Here's how the part is built. I have some questions about the finished solid (model axes, mm). Round coordinates to 2 decimals unless told otherwise and drop trailing zeros. Order: outer loops, then holes, each group sorted by start corner. A loop starts at its lowest first (then second) coordinate and runs counter-clockwise, first axis right, second up.
```python
from build123d import *

# Parameters (mm, degrees)
EXTRUDE_2_DEPTH    = 12
CHAMFER_1_SIZE     = 3
HOLE_WIZARD_M6_2_D = 5
F_8_0MM_1_D        = 8


with BuildPart() as part:
    # 草圖2 → 填料-伸長2 (new body)
    with BuildSketch(Plane(origin=(0, 0, 0), x_dir=(1, 0, 0), z_dir=(0, 1, 0))):
        Polygon((0, 86.602540378), (-75, 43.301270189), (-75, -43.301270189), (0, -86.602540378), (75, -43.301270189), (75, 43.301270189), align=None)
    extrude(amount=EXTRUDE_2_DEPTH)

    # 導角1
    chamfer_1_edges = [part.edges().sort_by_distance(p)[0] for p in [
        (-75, 12, 0),
        (-37.5, 12, 64.951905284),
        (37.5, 12, 64.951905284),
        (75, 12, 0),
        (37.5, 12, -64.951905284),
        (-37.5, 12, -64.951905284),
    ]]
    chamfer(chamfer_1_edges, length=CHAMFER_1_SIZE)

    # M6 螺紋孔2 (through all)
    with Locations(Plane(origin=(-65, 12, 37.527767497), x_dir=(0, 0, 1), z_dir=(0, 1, 0))):
        with Locations((0, 0), (-75.055534994, 0), (-112.583302492, 65), (-75.055534994, 130), (-37.527767497, 130), (37.527767498, 65), (0, 130)):
            Hole(HOLE_WIZARD_M6_2_D / 2)

    # Ø8.0mm 定位孔1 (through all)
    with Locations(Plane(origin=(-65, 12, 0), x_dir=(0, 0, 1), z_dir=(0, 1, 0))):
        with Locations((0, 0), (56.5, 32.5), (56.5, 97.5), (-56.5, 97.5), (-56.5, 32.5)):
            Hole(F_8_0MM_1_D / 2)


solid = part.part
```
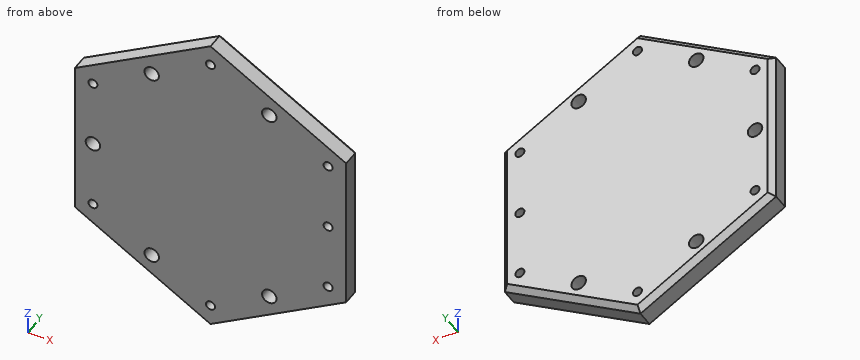
1. If we section it at A-A, the plane z = 0: Write out the boundary of the cut face in (x, y).
Evaluation:
outline: (-75, 0) - (-69, 0) - (-69, 12) - (-72, 12) - (-75, 9) - close; (-61, 0) - (62.5, 0) - (62.5, 12) - (-61, 12) - close; (67.5, 0) - (75, 0) - (75, 9) - (72, 12) - (67.5, 12) - close
2. I need wall thicknesses on probe 1 along X at (y, z) = (3.5, 0); probe 2 along X at (y, z) = (7, 54); probe 3 along Z at (x, y) = (-32, 8). Which ranges of each line are inside material? Lowest first, please.
Evaluation:
probe 1: x = -75 to -69, -61 to 62.5, 67.5 to 75
probe 2: x = -56.47 to -35.62, -29.38 to 29.38, 35.62 to 56.47
probe 3: z = -68.13 to -60.47, -52.53 to 52.53, 60.47 to 68.13
3. If we section it at C-C, the plane y = 5.5: State how many separate pieces and enclosed holes the cut face has, and give its area (3 significant figures).
Evaluation:
separate pieces: 1
enclosed holes: 12
area: 19,100 mm2
4. I'm going to push flat-ended pins straight in: P1, Ø4.5, axis at x = 0, z = -75.06, coming from the -Y side; P2, Ø4, axis at x = -6.5, y = 9.5, coming from the -Z side; P3, Ø6.5, axis at x = 65, z = 37.53, coming from the -Y side. Where does each tip first touch, or does it pass through?
Evaluation:
P1: passes through
P2: stops at z = -83.97
P3: stops at y = 0
5. If we section it at D-D, the plane x = 32.5: Write out the boundary of the cut face in (y, z).
Evaluation:
outline: (0, -67.84) - (9, -67.84) - (12, -64.37) - (12, -60.5) - (0, -60.5) - close; (0, -52.5) - (12, -52.5) - (12, 52.5) - (0, 52.5) - close; (0, 60.5) - (12, 60.5) - (12, 64.37) - (9, 67.84) - (0, 67.84) - close
6. If we section it at B-B, the plane x = -65: Write out the boundary of the cut face in (y, z), and give its area (3 significant figures).
Evaluation:
outline: (0, -49.07) - (9, -49.07) - (12, -45.61) - (12, -40.03) - (0, -40.03) - close; (0, -35.03) - (12, -35.03) - (12, -4) - (0, -4) - close; (0, 4) - (12, 4) - (12, 35.03) - (0, 35.03) - close; (0, 40.03) - (12, 40.03) - (12, 45.61) - (9, 49.07) - (0, 49.07) - close
area: 951 mm2
